Geometry check sheet. Reference: drawing and pictorial views, mm from the part's lowest x, y, z. A direction names the side the tool comes from. Round coordinates to 2 decimals unless told otherwise and drop trailing zeros. Order: outer loops, then holes, each group sorted by start corner. A loop starts at its lowest first (then second) coordinate and runs counter-clockwise, first axis right, second up.
(1) Tool access check on the marked faces 4 and 5. Record the directions out of +Z, -Z, +X, -X, +Y, -Y that give a thin tool (end or side, any length) a straight path to the whole face; none if there is none.
(2) Sectioned sample at B-B, the plane z = 5.5. Enter the section's corners in (x, y).
(3) Thickness scan on probe 1 along Z at (x, y) = (5.5, 6.25); probe 2 along X at (y, z) = (12.5, 8.75); probe 3 along Z at (x, y) = (3.75, 14.5) (1 decimal). Record the ranges inside material, lowest first.
(4) Mould release check, pull along Z, two halves, no side actions. Record for the marked faces 1, 2 and 3: released by +Z, released by -Z, zero draft, split by the parting line, or undercut.
(5) Sectioned sample at C-C, the plane y = 13. Enter the section's corners in (x, z) (1 decimal).
(6) Depth check by flat-ended pin: pin 1 (1.5 mm diameter, centred on x = 7, z = 2, fed in from -Y). Enter the tip coordinate at first touch or a pass-through.
(7) Sectioned sample at A-A, the plane y = 5.5. Enter the section's corners in (x, z).
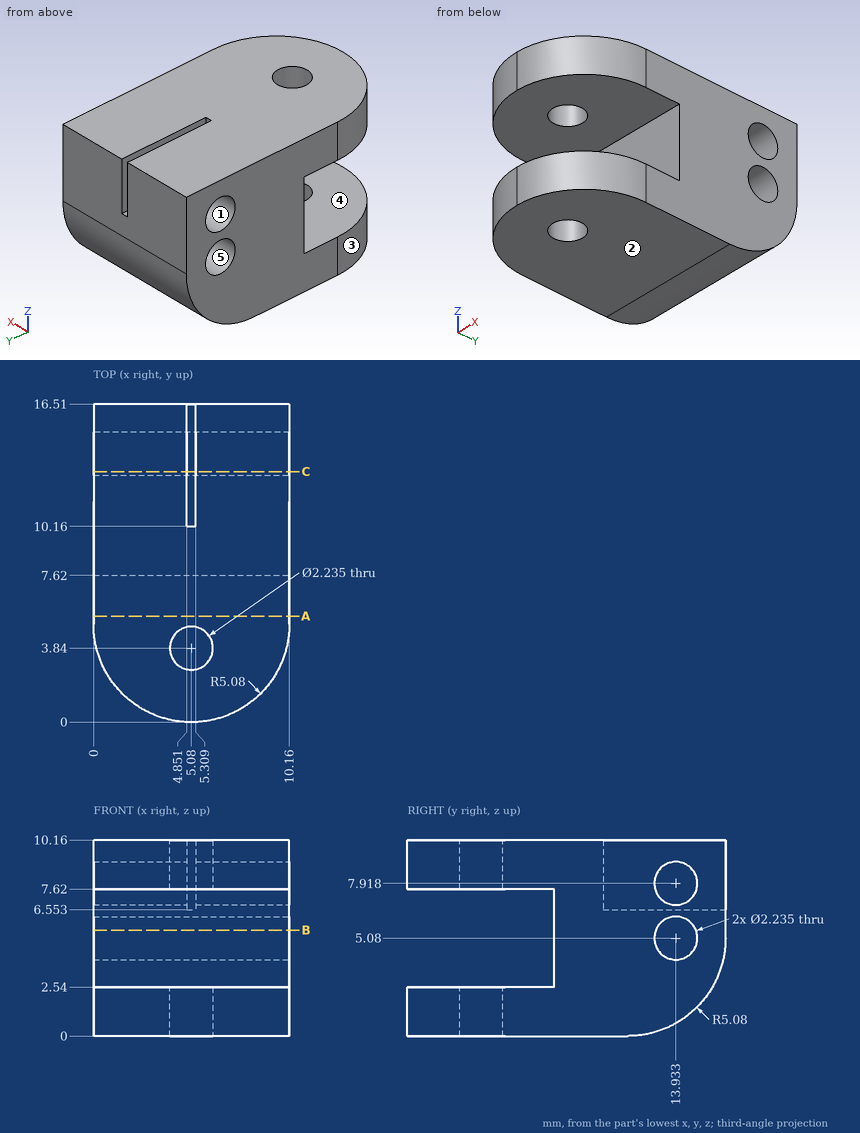
Derived:
1. face 4: +X, -X, -Y
1. face 5: +X, -X
2. outline: (0, 7.62) - (10.16, 7.62) - (10.16, 12.9) - (0, 12.9) - close; (0, 14.97) - (10.16, 14.97) - (10.16, 16.51) - (0, 16.51) - close
3. probe 1: z = 0 to 2.54, 7.62 to 10.16
3. probe 2: x = 0 to 4.85, 5.31 to 10.16
3. probe 3: z = 1 to 4.1, 6 to 7, 8.9 to 10.2
4. face 1: undercut
4. face 2: released by -Z
4. face 3: zero draft
5. outline: (0, 0.2) - (10.2, 0.2) - (10.2, 4.5) - (0, 4.5) - close; (0, 5.7) - (10.2, 5.7) - (10.2, 7.3) - (5.3, 7.3) - (5.3, 6.6) - (4.9, 6.6) - (4.9, 7.3) - (0, 7.3) - close; (0, 8.5) - (4.9, 8.5) - (4.9, 10.2) - (0, 10.2) - close; (5.3, 8.5) - (10.2, 8.5) - (10.2, 10.2) - (5.3, 10.2) - close
6. pin 1: stops at y = 0.14
7. outline: (0, 0) - (10.16, 0) - (10.16, 2.54) - (0, 2.54) - close; (0, 7.62) - (10.16, 7.62) - (10.16, 10.16) - (0, 10.16) - close
